Source: three-view drawing plus pictorial views. Frame: mm from the lowest corner of the part. A direction names the side the tool comes from. Give positions to 0.01 mm unless a question says otherwise; leave off trailing zeros. Order: outer loops, then holes, each group sorted by start corner. A loop starts at its lowest first (then second) coordinate and runs counter-clockwise, first axis right, second up. Notation, with made-up numbers: M -4.75,78 L 44.25,78 A32 cw 44.25,104 Z; hole C 70.5,43 d11. An arc over 180 degrees is marked long. Use CSV: the item, a comma, the result in double quotes. Start each with the question number.
Item 1: Access query for the marked faces 4 and 5. Directions: +Z, -Z, +X, -X, +Y, -Y. A direction counts if a zero-diameter tool reaches every point of the face in a straight line with its end or side. Return the directions, or none.
Item 2: First-contact query: pin 1 (4 mm diameter, centred on x = 26.5, y = 18, fed in from +Z) (1 decimal); pin 2 (4 mm diameter, centred on x = 26.5, z = 67.5, fed in from -Y); pin 3 (2 mm diameter, centred on y = 12, z = 41, fed in from -X); pin 4 (1.5 mm diameter, centred on y = 8, z = 55, fed in from +X) (1 decimal). Flat tips, straight axial feed; report the tip coordinate or a pass-through.
Item 3: Section query A-A on z = 73. Return loops of the section in (x, y) (1 decimal).
Item 4: Section query D-D on x = 38. Return loops of the section in (y, z) (1 decimal).
Item 5: Pull-direction query (Y, two-part tool) for the marked faces 1, 2 and 3; classes: +Y half, -Y half, draft (parallel to the pull), parting line (faces both ways), or undercut.
Item 6: Section query B-B on y = 28. Return loops of the section in (x, z) (1 decimal).
Item 7: Ray query, probe 1 along Y at (x, z) = (17, 65.5); probe 2 along Z at (x, y) = (43, 1.5) (1 decimal); probe 3 along X at (y, z) = (18.5, 58) (1 decimal). Return the intervals inside material, ascending. Write a range as from..to.
Item 8: Section query C-C on z = 54. Return loops of the section in (x, y) (1 decimal).
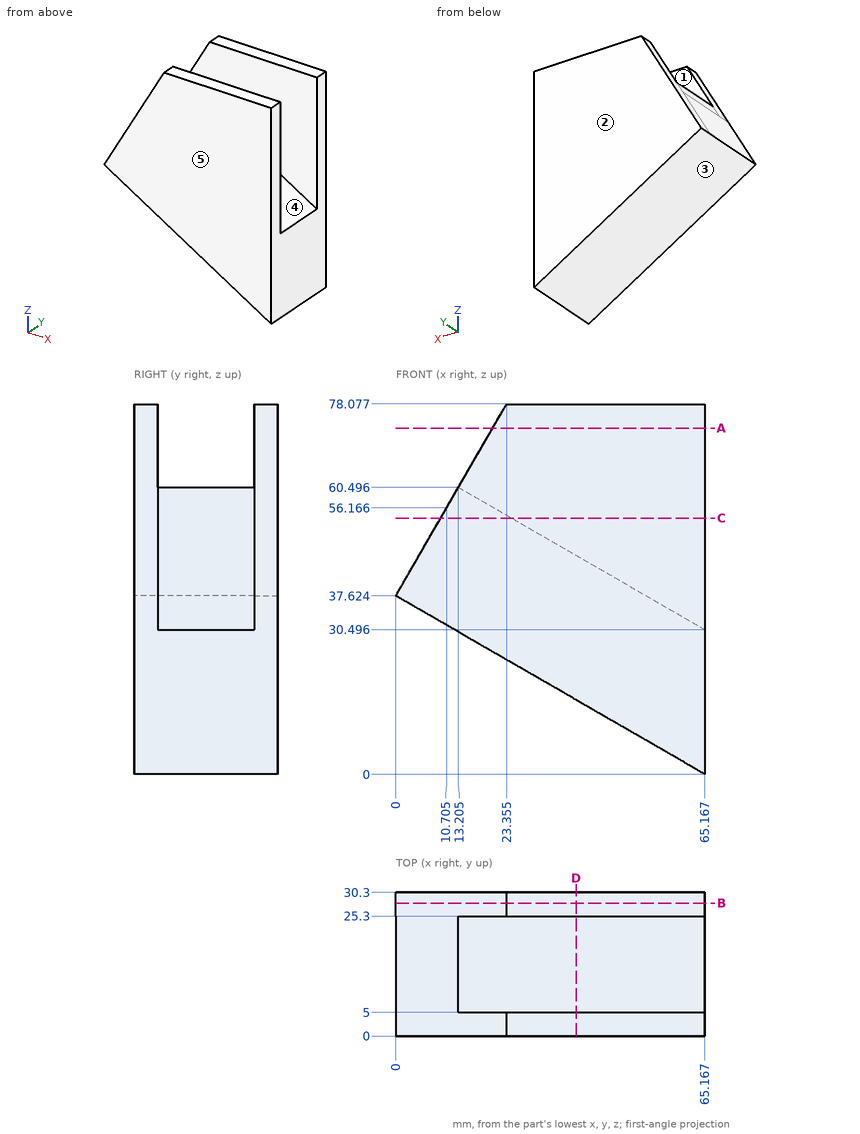
Verdict:
1,face 4,"+Z, +X"
1,face 5,"+Z, -Z, +X, -X, -Y"
2,pin 1,"z = 54"
2,pin 2,"y = 0"
2,pin 3,"x = 1.37"
2,pin 4,"x = 24"
3,outline,"M 20.4,0 L 65.2,0 L 65.2,5 L 20.4,5 Z; M 20.4,25.3 L 65.2,25.3 L 65.2,30.3 L 20.4,30.3 Z"
4,outline,"M 0,15.7 L 30.3,15.7 L 30.3,78.1 L 25.3,78.1 L 25.3,46.2 L 5,46.2 L 5,78.1 L 0,78.1 Z"
5,face 1,"undercut"
5,face 2,"+Y half"
5,face 3,"draft"
6,outline,"M 0,37.6 L 65.2,0 L 65.2,78.1 L 23.4,78.1 Z"
7,probe 1,"0..5, 25.3..30.3"
7,probe 2,"12.8..78.1"
7,probe 3,"11.8..17.5"
8,outline,"M 9.5,0 L 65.2,0 L 65.2,5 L 24.5,5 L 24.5,25.3 L 65.2,25.3 L 65.2,30.3 L 9.5,30.3 Z"
